```python
from build123d import *

# Parameters (mm, degrees)
SKETCH_1_W               = 100
SKETCH_1_H               = 85
EXTRUDE_1_DEPTH          = 15
EXTRUDE_2_DEPTH          = 15
EXTRUDE_START            = -27
SKETCH_3_W               = 42
SKETCH_3_H               = 42
EXTRUDE_3_DEPTH          = 12
CHAMFER_1_SIZE           = 3
EXTRUDE_START_2          = -15
EXTRUDE_4_DEPTH          = 15
SKETCH_6_R               = 27.5
EXTRUDE_5_DEPTH          = 23
SKETCH_7_R               = 24
EXTRUDE_6_DEPTH          = 7
SKETCH_8_R               = 12.5
EXTRUDE_7_DEPTH          = 7
SKETCH_9_R               = 9.5
CUT_EXTRUDE_1_DEPTH      = 15
SKETCH_11_R              = 27.5
EXTRUDE_9_DEPTH          = 2
CUT_EXTRUDE_2_DEPTH      = 39.5
CUT_EXTRUDE_2_DEPTH_BACK = 39.5
SKETCH_12_R              = 12.05
SKETCH_13_R              = 7.5
CUT_EXTRUDE_3_DEPTH      = 120.787311515
CHAMFER_2_SIZE           = 2
CHAMFER_3_SIZE           = 2
CUT_EXTRUDE_START        = -3.5
SKETCH_10_R              = 39
SKETCH_10_R_2            = 27.5
CUT_EXTRUDE_4_DEPTH      = 3.5
SKETCH_15_R              = 1.65
CUT_EXTRUDE_5_DEPTH      = 97.124918726
SKETCH_16_W              = 105.441549674
SKETCH_16_H              = 43.677503156
CUT_EXTRUDE_6_DEPTH      = 120.787311515
CUT_EXTRUDE_7_DEPTH      = 95.5
CUT_EXTRUDE_7_DEPTH_BACK = 95.5
SKETCH_17_R              = 2.15
SKETCH_18_R              = 4
CUT_EXTRUDE_8_DEPTH      = 3
CUT_EXTRUDE_9_DEPTH      = 85.351941294
SKETCH_20_R              = 11.1
CUT_EXTRUDE_10_DEPTH     = 2.1
EXTRUDE_START_3          = -12
EXTRUDE_10_DEPTH         = 18


with BuildPart() as part:
    # 草图1 → 凸台-拉伸1 (new body)
    with BuildSketch(Plane(origin=(0, 0, 0), x_dir=(1, 0, 0), z_dir=(0, 1, 0))):
        Rectangle(SKETCH_1_W, SKETCH_1_H)
    extrude(amount=EXTRUDE_1_DEPTH)

    # 草图2 → 凸台-拉伸2 (add)
    with BuildSketch(Plane.XY.offset(42.5)):
        with BuildLine():
            Line((-50, 15), (-50, 47))
            ThreePointArc((-50, 47), (-33.100173908, 67.595838753), (-9.601088198, 55.042525778))
            Line((-9.601088198, 55.042525778), (7, 15))
            Line((7, 15), (-50, 15))
        make_face()
    extrude(amount=-EXTRUDE_2_DEPTH)

    # 草图3 → 凸台-拉伸3 (add)
    with BuildSketch(Plane(origin=(0, 0, -42.5), x_dir=(-1, 0, 0), z_dir=(0, 0, -1)).offset(EXTRUDE_START)):
        with Locations((-29, 36)):
            Rectangle(SKETCH_3_W, SKETCH_3_H)
    extrude(amount=-EXTRUDE_3_DEPTH)

    # 倒角1
    chamfer_1_edges = [part.edges().sort_by_distance(p)[0] for p in [
        (50, 57, -9.5),
        (8, 57, -9.5),
    ]]
    chamfer(chamfer_1_edges, length=CHAMFER_1_SIZE)

    # 草图5 → 凸台-拉伸4 (add)
    with BuildSketch(Plane(origin=(0, 0, -42.5), x_dir=(-1, 0, 0), z_dir=(0, 0, -1)).offset(EXTRUDE_START_2)):
        with BuildLine():
            Line((-7, 15), (50, 15))
            Line((50, 15), (50, 47))
            ThreePointArc((50, 47), (33.100173908, 67.595838753), (9.601088198, 55.042525778))
            Line((9.601088198, 55.042525778), (-7, 15))
        make_face()
    extrude(amount=EXTRUDE_4_DEPTH)

    # 草图6 → 凸台-拉伸5 (add)
    with BuildSketch(Plane.XZ):
        with Locations(Location((0, 0, 0), (0, 0, 270))):
            Circle(SKETCH_6_R)
    extrude(amount=EXTRUDE_5_DEPTH)

    # 草图7 → 凸台-拉伸6 (add)
    with BuildSketch(Plane.XZ.offset(23)):
        with Locations(Location((0, 0, 0), (0, 0, 270))):
            Circle(SKETCH_7_R)
    extrude(amount=EXTRUDE_6_DEPTH)

    # 草图8 → 凸台-拉伸7 (add)
    with BuildSketch(Plane.XZ.offset(30)):
        with Locations(Location((0, 0, 0), (0, 0, 270))):
            Circle(SKETCH_8_R)
    extrude(amount=EXTRUDE_7_DEPTH)

    # 草图9 → 切除-拉伸1 (cut)
    with BuildSketch(Plane(origin=(0, 0, -15.5), x_dir=(-1, 0, 0), z_dir=(0, 0, -1))):
        with Locations((-29, 36)):
            Circle(SKETCH_9_R)
    extrude(amount=-CUT_EXTRUDE_1_DEPTH, mode=Mode.SUBTRACT)

    # 草图11 → 凸台-拉伸9 (add)
    with BuildSketch(Plane.XZ.offset(30)):
        with Locations(Location((0, 0, 0), (0, 0, 270))):
            Circle(SKETCH_11_R)
    extrude(amount=EXTRUDE_9_DEPTH)

    # 草图12 → 切除-拉伸2 (cut, two sides: drawn at the far end of the back side and taken through both)
    with BuildSketch(Plane.XY.offset(-CUT_EXTRUDE_2_DEPTH_BACK)):
        with Locations(Location((-29, 47, 0), (0, 0, 180))):
            Circle(SKETCH_12_R)
    extrude(amount=CUT_EXTRUDE_2_DEPTH + CUT_EXTRUDE_2_DEPTH_BACK, mode=Mode.SUBTRACT)

    # 草图13 → 切除-拉伸3 (cut, through all)
    with BuildSketch(Plane.XY.offset(42.5)):
        with Locations((-29, 47)):
            Circle(SKETCH_13_R)
    extrude(amount=-CUT_EXTRUDE_3_DEPTH, mode=Mode.SUBTRACT)

    # 倒角2
    chamfer_2_edges = [part.edges().sort_by_distance(p)[0] for p in [
        (-36.5, 47, 42.5),
        (28.5, 15, 42.5),
        (-1.300544099, 35.021262889, 42.5),
        (-33.100173908, 67.595838753, 42.5),
        (0, 0, 42.5),
        (50, 7.5, 42.5),
        (-50, 23.5, 42.5),
    ]]
    chamfer(chamfer_2_edges, length=CHAMFER_2_SIZE)

    # 倒角3
    chamfer_3_edges = [part.edges().sort_by_distance(p)[0] for p in [
        (0, 0, -42.5),
        (-1.300544099, 35.021262889, -42.5),
        (-33.100173908, 67.595838753, -42.5),
        (28.5, 15, -42.5),
        (-50, 23.5, -42.5),
        (50, 7.5, -42.5),
        (-36.5, 47, -42.5),
    ]]
    chamfer(chamfer_3_edges, length=CHAMFER_3_SIZE)

    # 草图10 → 切除-拉伸4 (cut)
    with BuildSketch(Plane.XZ.offset(CUT_EXTRUDE_START)):
        with Locations(Location((0, 0, 0), (0, 0, 270))):
            Circle(SKETCH_10_R)
        with Locations(Location((0, 0, 0), (0, 0, 270))):
            Circle(SKETCH_10_R_2, mode=Mode.SUBTRACT)
    extrude(amount=CUT_EXTRUDE_4_DEPTH, mode=Mode.SUBTRACT)

    # 草图15 → 切除-拉伸5 (cut, through all)
    with BuildSketch(Plane.XY.offset(-3.5)):
        with Locations((44.5, 51.5)):
            Circle(SKETCH_15_R)
        with Locations((13.5, 51.5)):
            Circle(SKETCH_15_R)
        with Locations((13.5, 20.5)):
            Circle(SKETCH_15_R)
        with Locations((44.5, 20.5)):
            Circle(SKETCH_15_R)
    extrude(amount=-CUT_EXTRUDE_5_DEPTH, mode=Mode.SUBTRACT)

    # 草图16 → 切除-拉伸6 (cut, through all)
    with BuildSketch(Plane(origin=(0, 0, -42.5), x_dir=(-1, 0, 0), z_dir=(0, 0, -1))):
        with Locations((2.720774837, -21.838751578)):
            Rectangle(SKETCH_16_W, SKETCH_16_H)
    extrude(amount=-CUT_EXTRUDE_6_DEPTH, mode=Mode.SUBTRACT)

    # 草图17 → 切除-拉伸7 (cut, two sides: drawn at the far end of the back side and taken through both)
    with BuildSketch(Plane(origin=(0, 0, 0), x_dir=(1, 0, 0), z_dir=(0, 1, 0)).offset(-CUT_EXTRUDE_7_DEPTH_BACK)):
        with Locations(Location((-2.898938749, -15.735188405, 0), (0, 0, 90))):
            Circle(SKETCH_17_R)
        with Locations(Location((-15.735188405, 2.898938749, 0), (0, 0, 90))):
            Circle(SKETCH_17_R)
        with Locations(Location((2.898938749, 15.735188405, 0), (0, 0, 90))):
            Circle(SKETCH_17_R)
        with Locations(Location((15.735188405, -2.898938749, 0), (0, 0, 90))):
            Circle(SKETCH_17_R)
    extrude(amount=CUT_EXTRUDE_7_DEPTH + CUT_EXTRUDE_7_DEPTH_BACK, mode=Mode.SUBTRACT)

    # 草图18 → 切除-拉伸8 (cut)
    with BuildSketch(Plane(origin=(0, 15, 0), x_dir=(1, 0, 0), z_dir=(0, 1, 0))):
        with Locations(Location((2.898938749, 15.735188405, 0), (0, 0, 270))):
            Circle(SKETCH_18_R)
        with Locations(Location((15.735188405, -2.898938749, 0), (0, 0, 270))):
            Circle(SKETCH_18_R)
        with Locations(Location((-2.898938749, -15.735188405, 0), (0, 0, 270))):
            Circle(SKETCH_18_R)
        with Locations(Location((-15.735188405, 2.898938749, 0), (0, 0, 270))):
            Circle(SKETCH_18_R)
    extrude(amount=-CUT_EXTRUDE_8_DEPTH, mode=Mode.SUBTRACT)

    # 草图19 → 切除-拉伸9 (cut, through all)
    with BuildSketch(Plane(origin=(0, 15, 0), x_dir=(1, 0, 0), z_dir=(0, 1, 0))):
        with BuildLine():
            Line((-2.664582519, 3.05), (2.664582519, 3.05))
            ThreePointArc((2.664582519, 3.05), (0, -4.05), (-2.664582519, 3.05))
        make_face()
    extrude(amount=-CUT_EXTRUDE_9_DEPTH, mode=Mode.SUBTRACT)

    # 草图20 → 切除-拉伸10 (cut)
    with BuildSketch(Plane.XY.offset(-3.5)):
        with Locations((29, 36)):
            Circle(SKETCH_20_R)
    extrude(amount=-CUT_EXTRUDE_10_DEPTH, mode=Mode.SUBTRACT)

    # 草图21 → 凸台-拉伸10 (add)
    with BuildSketch(Plane(origin=(50, 0, 0), x_dir=(0, 0, -1), z_dir=(1, 0, 0)).offset(EXTRUDE_START_3)):
        Polygon((15.5, 25), (15.5, 15), (25.5, 15), align=None)
    extrude(amount=-EXTRUDE_10_DEPTH)


solid = part.part
```
Model file for the job. Use its own axes, mm. A direction names the side the tool comes from. Give positions to 0.01 mm unless a question says otherwise; leave off trailing zeros. Write each loop counter-clockwise with the first axis right and the second up, starting at its lowest first coordinate (ties: lowest second). Pieces come first, ordered by that corner, then holes. Notation, with made-up numbers: (38.25, 79) -> (71.25, 79) arc R17 cw to (71.25, 112) -> close; hole circle Ø10 at (37, 30). An arc over 180 degrees is marked (long way). Use CSV: the item, a comma, the result in double quotes. Start each with the question number.
1) Two-plate mould, pull along X, no slides. Class faces 1 (the flat face through (38, 18, -18)), 2 (the flat face through (29.1, 19.9, -20.6)), 3 (the cylindrical face through (14.39, 52.89, -9.42)): released by +X, released by -X, zero draft, split by the parting line, or undercut.
2) Cut at A-A on x = 44.5. List the corners of the cut face in (y, z), plus the area to 3 significant figures.
3) Tool access for faces 4 (the flat face through (-23, 52, -39.5)), 5 (the flat face through (8, 34, -10)), 6 (the flat face through (-21, 36, -27.5)): list every direction of +Z, -Z, +X, -X, +Y, -Y with a clear straight run to the whole face (end or side of a thin tool).
4) Cut at B-B on y = 16.5. List the corners of the cut face in (x, z).
5) Cut at C-C on x = 29. List the corners of the cut face in (y, z), plus the area to 3 significant figures.
6) Pin check, flat tips, straight feed: P1, Ø12, axis at x = -27.5, y = 49, coming from the -Z side; P2, Ø10.5, axis at x = 0, z = 0, coming from the +Y side; P3, Ø2.5, axis at x = -4.5, z = 16, coming from the +Y side. Stop position of each tip, or through.
7) Cut at D-D on y = 51.5. Count the separate pieces of the cut face and the enclosed holes in it, plus the area to 3 significant figures.
8) Drill centre lines: L1, parallel to Y at x = 13.5, z = -7.25; L2, parallel to Y at x = -29, z = 40.25; L3, parallel to Y at x = -29, z = -36. Where is each one in solid material? Low to high.
Final values:
1,face 1,"released by +X"
1,face 2,"zero draft"
1,face 3,"undercut"
2,outline,"(0, -40.5) -> (2, -42.5) -> (13, -42.5) -> (15, -40.5) -> (15, -15.5) -> (18.85, -15.5) -> (18.85, -3.5) -> (15, -3.5) -> (15, 40.5) -> (13, 42.5) -> (2, 42.5) -> (0, 40.5) -> close; (22.15, -15.5) -> (49.85, -15.5) -> (49.85, -3.5) -> (22.15, -3.5) -> close; (53.15, -15.5) -> (57, -15.5) -> (57, -3.5) -> (53.15, -3.5) -> close"
2,area,"1,690 mm2"
3,face 4,"none"
3,face 5,"+Z, -Z, -X, +Y"
3,face 6,"+X, -X, +Y"
4,outline,"(-50, -40.5) -> (-48, -42.5) -> (4.21, -42.5) -> (6.38, -40.5) -> (6.38, -27.5) -> (-50, -27.5) -> close; (-50, 27.5) -> (6.38, 27.5) -> (6.38, 40.5) -> (4.21, 42.5) -> (-48, 42.5) -> (-50, 40.5) -> close; (8, -15.5) -> (20, -15.5) -> (20, -24) -> (38, -24) -> (38, -15.5) -> (50, -15.5) -> (50, -3.5) -> (8, -3.5) -> close"
5,outline,"(0, -40.5) -> (2, -42.5) -> (13, -42.5) -> (15, -40.5) -> (15, -25.5) -> (25, -15.5) -> (26.5, -15.5) -> (26.5, -5.6) -> (24.9, -5.6) -> (24.9, -3.5) -> (15, -3.5) -> (15, 40.5) -> (13, 42.5) -> (2, 42.5) -> (0, 40.5) -> (0, 26.08) -> (3.5, 26.08) -> (3.5, -26.08) -> (0, -26.08) -> close; (45.5, -15.5) -> (57, -15.5) -> (57, -3.5) -> (47.1, -3.5) -> (47.1, -5.6) -> (45.5, -5.6) -> close"
5,area,"1,400 mm2"
6,P1,"stops at z = -41.5"
6,P2,"stops at y = 15"
6,P3,"stops at y = 12"
7,separate pieces,"7"
7,enclosed holes,"0"
7,area,"1,040 mm2"
8,L1,"y = 0 to 18.85, 22.15 to 49.85, 53.15 to 57"
8,L2,"y = 0 to 39.5, 54.5 to 68"
8,L3,"y = 0 to 34.95, 59.05 to 68"
